The drawing under review shows one solid part. Ordinate dimensions are in mm from its lowest x, y, z. A direction names the side the tool comes from. Coordinates: 2 decimals unless noted, no trailing zeros. Write each loop counter-clockwise with the first axis right and the second up, starting at its lowest first coordinate (ties: lowest second). Pieces come first, ordered by that corner, then holes. Notation, with made-up numbers: (38.5, 17) - (75.5, 17) arc R19 ccw to (75.5, 29) - close; hole circle Ø10 at (88.25, 1.25). An arc over 180 degrees is marked (long way). Put each result on its own line as item: value. Start each with the question number.
Item 1: Consider section B-B on y = 35. Give the boundary of the cut face in (x, z) (1 decimal).
Item 2: Machinability: for the marked faces 1 and 2, which of the approach directions +Z, -Z, +X, -X, +Y, -Y give a long, thin tool a straight path to every point of the face, cutting with its end or side? Answer none if there is none.
Item 3: Consider section C-C on z = 30.5. Give the boundary of the cut face in (x, y).
Item 4: To check wall thickness, follow L1, parallel to Z at x = 16.5, y = 35 (1 decimal); L2, parallel to Y at x = 29, z = 33.5. State the ranges of each line that lie inside material, in increasing order. Write a range as [from, to].
Item 5: For pin 1 (8 mm diameter, centred on x = 10.5, z = 13.5, fed in from +Y), flat-tipped, find the tip position at first contact; note if it passes through.
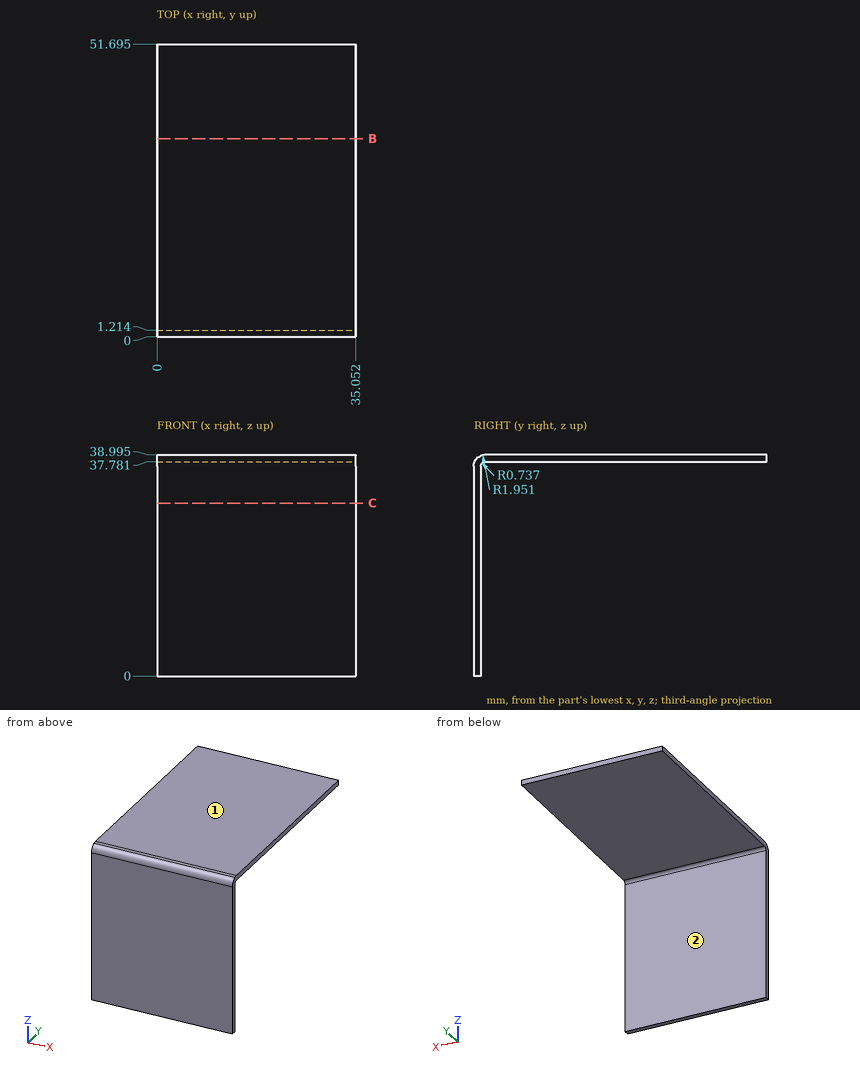
Report:
1. outline: (0, 37.8) - (35.1, 37.8) - (35.1, 39) - (0, 39) - close
2. face 1: +Z, +X, -X, +Y, -Y
2. face 2: -Z, +X, -X, +Y
3. outline: (0, 0) - (35.05, 0) - (35.05, 1.21) - (0, 1.21) - close
4. L1: [37.8, 39]
4. L2: [0, 1.21]
5. pin 1: y = 1.21
